Design review of the part built by this model. Coordinates are the model's own, in mm. A direction names the side the tool comes from. Give positions to 0.01 mm unless a question says otherwise; leave off trailing zeros. Write each loop counter-clockwise with the first axis right and the second up, starting at its lowest first coordinate (ties: lowest second). Pieces come first, ordered by that corner, then holes. Notation, with made-up numbers: (-29, -35.5) -> (-19, -35.5) arc R20 cw to (-19, -27.5) -> close; hole circle Ø6 at (-25.75, 37). An arc over 180 degrees is marked (long way). Write each question's results on one line, items separated by ' | '. Start each with the question number.
(1) Take a section at D-D (z = -7.5). State the section outline as (x, y) points, plus the area to 3 significant figures.
(2) Take a section at A-A (x = -9). State the section outline as (y, z) points.
(3) Mouldability with a two-part tool opening along X and no side actions: class faces 1 (the face through (0, 15, 25)), 2 (the face through (21.99, 15.21, 22.15)), 3 (the face through (-17.93, 4.93, -14.35)), 4 (the face through (-25, 15, 0)) as released by +X, released by -X, zero draft, split by the parting line, or undercut.
(4) For faces 5 (the face through (0, 10, 0)), 6 (the face through (15, 10, -15)), 7 (the face through (21.99, 15.21, -22.15)), list the 3-axis set-ups (+Z, -Z, +X, -X, +Y, -Y) from which the entire face can be reached by the end or side of a thin tool; tool diameter is ignored.
(5) To check wall thickness, follow probe 1 along X at (y, z) = (5.5, -15); probe 2 along X at (y, z) = (20.5, 9); probe 3 along Z at (x, y) = (17, 9). State the ranges of each line that lie inside material, in increasing order.
(6) Clearance check with flat-ended pins moving along their axes: pin 1 (5.5 mm diameter, centred on x = 15, z = -15, fed in from -Y); pin 2 (3 mm diameter, centred on y = 18.5, z = -19, fed in from -X); pin 3 (9 mm diameter, centred on x = -3, z = 7, fed in from +Y). State where each tip first meets the part, or that it passes through.
(7) Take a section at C-C (y = 3). State the section outline as (x, z) points.
(8) Take a section at B-B (y = 15.25). State the section outline as (x, z) points, plus the area to 3 significant figures.
from build123d import *

# Parameters (mm, degrees)
SKETCH1_W           = 50
SKETCH1_H           = 50
BOSS_EXTRUDE1_DEPTH = 30
SKETCH2_R           = 15
CUT_EXTRUDE1_DEPTH  = 20
FILLET1_R           = 10
SKETCH3_R           = 3
CUT_EXTRUDE2_DEPTH  = 10


with BuildPart() as part:
    # Sketch1 → Boss-Extrude1 (new body)
    with BuildSketch(Plane(origin=(0, 0, 0), x_dir=(1, 0, 0), z_dir=(0, 1, 0))):
        Rectangle(SKETCH1_W, SKETCH1_H)
    extrude(amount=BOSS_EXTRUDE1_DEPTH)

    # Sketch2 → Cut-Extrude1 (cut)
    with BuildSketch(Plane(origin=(0, 30, 0), x_dir=(1, 0, 0), z_dir=(0, 1, 0))):
        with Locations(Location((0, 0, 0), (0, 0, 270))):
            Circle(SKETCH2_R)
    extrude(amount=-CUT_EXTRUDE1_DEPTH, mode=Mode.SUBTRACT)

    # Fillet1
    fillet1_edges = [part.edges().sort_by_distance(p)[0] for p in [
        (25, 15, 25),
        (-25, 15, 25),
        (-25, 15, -25),
        (25, 15, -25),
    ]]
    fillet(fillet1_edges, radius=FILLET1_R)

    # Sketch3 → Cut-Extrude2 (cut)
    with BuildSketch(Plane.XZ):
        with Locations(Location((15, -15, 0), (0, 0, 270))):
            Circle(SKETCH3_R)
        with Locations(Location((-15, -15, 0), (0, 0, 270))):
            Circle(SKETCH3_R)
        with Locations(Location((-15, 15, 0), (0, 0, 270))):
            Circle(SKETCH3_R)
        with Locations(Location((15, 15, 0), (0, 0, 270))):
            Circle(SKETCH3_R)
    extrude(amount=-CUT_EXTRUDE2_DEPTH, mode=Mode.SUBTRACT)


solid = part.part
Report:
1) outline: (-25, 0) -> (25, 0) -> (25, 30) -> (12.99, 30) -> (12.99, 10) -> (-12.99, 10) -> (-12.99, 30) -> (-25, 30) -> close | area: 980 mm2
2) outline: (0, -25) -> (30, -25) -> (30, -12) -> (10, -12) -> (10, 12) -> (30, 12) -> (30, 25) -> (0, 25) -> close
3) face 1: zero draft | face 2: released by +X | face 3: undercut | face 4: released by -X
4) face 5: +Y | face 6: -Y | face 7: -Z, +X, +Y, -Y
5) probe 1: -25 to -18, -12 to 12, 18 to 25 | probe 2: -25 to -12, 12 to 25 | probe 3: -24.8 to -17.24, -12.76 to 12.76, 17.24 to 24.8
6) pin 1: y = 10 | pin 2: x = -24.68 | pin 3: y = 10
7) outline: (-25, -15) arc R10 ccw to (-15, -25) -> (15, -25) arc R10 ccw to (25, -15) -> (25, 15) arc R10 ccw to (15, 25) -> (-15, 25) arc R10 ccw to (-25, 15) -> close; hole circle Ø6 at (-15, -15); hole circle Ø6 at (-15, 15); hole circle Ø6 at (15, -15); hole circle Ø6 at (15, 15)
8) outline: (-25, -15) arc R10 ccw to (-15, -25) -> (15, -25) arc R10 ccw to (25, -15) -> (25, 15) arc R10 ccw to (15, 25) -> (-15, 25) arc R10 ccw to (-25, 15) -> close; hole circle Ø30 at (0, 0) | area: 1,710 mm2
